Source: CAD feature listing. Evaluate the final solid. Frame: model axes, mm. Give positions to 0.01 mm unless a question says otherwise; leave off trailing zeros. Write each loop counter-clockwise with the first axis right and the second up, starting at its lowest first coordinate (ties: lowest second). Pieces come first, ordered by that corner, then holes. Notation, with made-up numbers: M 71.5,17.25 L 80.5,17.25 A25 ccw 80.5,56.25 Z; hole C -22,30 d5. An arc over 180 degrees is marked long. Return JSON: item names as keys, results as strings.
Autodesk Inventor part; units mm, degrees
ref_plane "YZ Plane" through (0, 0, 0) normal (1, 0, 0) x (0, 1, 0)
ref_plane "XZ Plane" through (0, 0, 0) normal (0, 1, 0) x (-1, 0, 0)
ref_plane "XY Plane" through (0, 0, 0) normal (0, 0, 1) x (1, 0, 0)
sketch "Sketch1" plane through (0, 0, 0) normal (0, 0, 1) x (1, 0, 0)
  line L0 (0, 0) -> (-7, 0) construction
  line L1 (-7, 0) -> (-7, 5)
  arc A0 (0, 12) -> (-7, 5) centre (0, 5) ccw
  line L2 (0, 12) -> (0, 0)
  line L3 (-7, 0) -> (-7, -5)
  arc A1 (-7, -5) -> (0, -12) centre (0, -5) ccw
  line L4 (0, -12) -> (0, 0)
  dimension "d0" = 7
  dimension "d2" = 7
  dimension "d5" = 5
extrude "Extrusion1" add sketch "Sketch1" along normal blind 3.175
properties part number "waterbottle_holder_side"
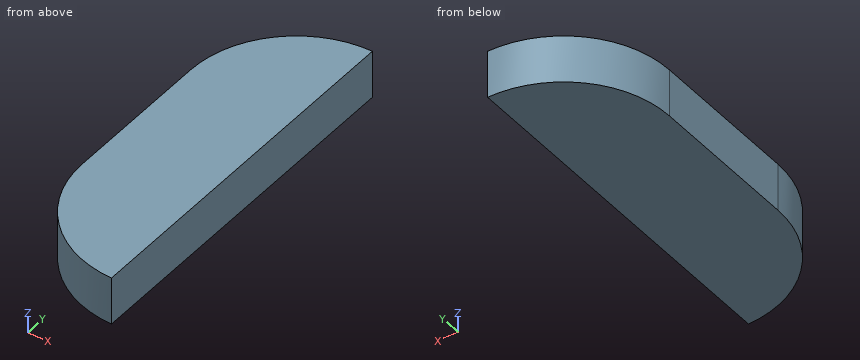
1) Cut plane B-B, the plane x = -3. Return the cut outline in (y, z) (3 decimals).
Numbers:
{"outline": "M -11.325,0 L 11.325,0 L 11.325,3.175 L -11.325,3.175 Z"}
2) Line query: line 1 (Y direction, x = -4, z = 1.45); line 2 (X direction, y = 10.5, z = 1.65); line 3 (Y direction, x = -6, z = 1.65). Output: solid intervals per line, ascending. Write a range as [from, to].
Numbers:
{"line 1": "y = [-10.74, 10.74]", "line 2": "x = [-4.33, 0]", "line 3": "y = [-8.61, 8.61]"}
3) Cut plane A-A, the plane z = 2.2. Return the cut outline in (x, y), then the cut area to 3 significant figures.
Numbers:
{"outline": "M -7,-5 A7 ccw 0,-12 L 0,12 A7 ccw -7,5 Z", "area": "147 mm²"}
4) Contact query for a flat-ended pin moving along its axis: pin 1 Ø1.5 at (x, z) = (-3.5, 2.5) entering from +Y. Output: stop coordinate, or through.
Numbers:
{"pin 1": "stops at y = 11.44"}
